Autodesk Inventor part; units mm, degrees
ref_plane "YZ Plane" through (0, 0, 0) normal (1, 0, 0) x (0, 1, 0)
ref_plane "XZ Plane" through (0, 0, 0) normal (0, 1, 0) x (-1, 0, 0)
ref_plane "XY Plane" through (0, 0, 0) normal (0, 0, 1) x (1, 0, 0)
ref_plane "工作平面1" through (0, 0, 214.75) normal (0, 0, 1) x (1, 0, 0)
sketch "草图2" plane through (0, 0, 214.75) normal (0, 0, 1) x (1, 0, 0)
  line L0 (15, -0.25) -> (15, -3.75)
  line L1 (15, 3.75) -> (15, 0.75)
  line L2 (15, 0.75) -> (13.5, 0.75)
  line L3 (13.5, 0.75) -> (13.5, -0.25)
  line L4 (13.5, -0.25) -> (15, -0.25)
  line L5 (27.5, 3.75) -> (-27.5, 3.75)
  line L6 (-15, 0.75) -> (-15, 3.75)
  line L7 (-15, -3.75) -> (-15, -0.25)
  line L8 (-13.5, 0.75) -> (-15, 0.75)
  line L9 (-13.5, -0.25) -> (-13.5, 0.75)
  line L10 (-15, -0.25) -> (-13.5, -0.25)
  line L11 (-15, -4.25) -> (15, -4.25)
  line L12 (-15, -3.75) -> (-15, -4.25)
  line L13 (15, -4.25) -> (15, -3.75)
  line L14 (18, 3.75) -> (18, -8.25)
  line L15 (-18, 3.75) -> (-18, -8.25)
  line L16 (-18, -8.25) -> (18, -8.25)
  point P0 (0, 0)
  dimension "d0" = 12
  dimension "d1" = 3
  dimension "d2" = 12
  dimension "d3" = 3
extrude "拉伸1" add sketch "草图2" along normal blind 50 contours L4 L3 L2 L1 L5 L14 L16 L15 L6 L8 L9 L10 L7 L12 L11 L13 L0
sketch "草图3" plane through (-18, -8.25, 214.75) normal (0, -1, 0) x (1, 0, 0)
  line L0 (0, 0) -> (0, 50)
  line L1 (0, 0) -> (36, 0)
  line L2 (0, 50) -> (14, 50)
  line L3 (14, 50) -> (14, 0)
  line L4 (14, 0) -> (0, 0)
  line L5 (0, 0) -> (0, 50)
  line L6 (0, 50) -> (36, 50)
  line L7 (36, 50) -> (22, 50)
  line L8 (22, 50) -> (22, 0)
  line L9 (22, 0) -> (36, 0)
  line L10 (36, 0) -> (36, 50)
  point P0 (18, -214.75)
  dimension "d6" = 14
  dimension "d7" = 14
extrude "拉伸2" add sketch "草图3" along normal blind 2 contours L0 L2 L3 L1 | L8 L6 L10 L1
sketch "草图4" plane through (-18, -10.25, 214.75) normal (0, -1, 0) x (1, 0, 0)
  line L0 (0, 50) -> (0, 0)
  line L1 (14, 50) -> (0, 50)
  line L2 (0, 0) -> (14, 0)
  line L3 (36, 50) -> (22, 50)
  line L4 (36, 0) -> (36, 50)
  line L5 (22, 0) -> (36, 0)
  point P0 (18, -214.75)
  point P1 (7, 42)
  point P2 (7, 8)
  point P3 (29, 42)
  point P4 (29, 8)
  dimension "d10" = 7
  dimension "d11" = 8
  dimension "d12" = 8
  dimension "d13" = 7
  dimension "d14" = 8
  dimension "d15" = 7
  dimension "d16" = 7
  dimension "d17" = 8
hole "孔1" at (-11, -10.25, 256.75) at (-11, -10.25, 222.75) at (11, -10.25, 256.75) at (11, -10.25, 222.75) direction (0, 1, 0) diameter 3.242 depth 3 tip angle 118
properties part number "滑块"
Read the model definition and answer for the solid it produces. Units are mm, in the model's axes. A direction names the side the tool comes from. Coordinates: 2 decimals unless noted, no trailing zeros. Loops run counter-clockwise (first coordinate to the right, second up) from the corner with the lowest first, then second, coordinate; pieces in that order, holes last. Notation, with made-up numbers: (9, -15.75) -> (23, -15.75) arc R31 ccw to (23, 20.25) -> close; hole circle Ø6 at (88, -36.5). An arc over 180 degrees is marked (long way). Return JSON: item names as keys, results as strings.
Item 1: For a pull along X with two mould halves and no side action, classify faces 6 (the flat face through (0, -5, 214.75)), 7 (the cylindrical face through (-11.07, -8.73, 224.37)), 8 (the flat face through (-15, -2, 239)) as +X half, -X half, draft (parallel to the pull), parting line (faces both ways), or undercut.
Answers:
{"face 6": "draft", "face 7": "undercut", "face 8": "undercut"}
Item 2: Find section C-C (x = 3). Determine the outline of the cut face in (y, z).
Answers:
{"outline": "(-8.25, 214.75) -> (-4.25, 214.75) -> (-4.25, 264.75) -> (-8.25, 264.75) -> close"}
Item 3: Flat-ended cylindrical pins translate along their axes: P1, Ø3, axis at x = 11, z = 222.75, coming from the +Y side; P2, Ø6, axis at x = 11, z = 252.5, coming from the +Y side; P3, Ø2, axis at x = 10.5, y = -3, coming from the +Z side. Find the tip coordinate at first contact, or state that the pin passes through.
Answers:
{"P1": "stops at y = -4.25", "P2": "stops at y = 0.75", "P3": "passes through"}
Item 4: Find section B-B (z = 231). Determine the outline of the cut face in (x, y).
Answers:
{"outline": "(-18, -10.25) -> (-4, -10.25) -> (-4, -8.25) -> (4, -8.25) -> (4, -10.25) -> (18, -10.25) -> (18, 3.75) -> (15, 3.75) -> (15, 0.75) -> (13.5, 0.75) -> (13.5, -0.25) -> (15, -0.25) -> (15, -4.25) -> (-15, -4.25) -> (-15, -0.25) -> (-13.5, -0.25) -> (-13.5, 0.75) -> (-15, 0.75) -> (-15, 3.75) -> (-18, 3.75) -> close"}
Item 5: Find the intervals of material crossed by probe 1 along X at (y, z) = (-8.9, 222.75); probe 2 along Z at (x, y) = (-11, -9); probe 3 along X at (y, z) = (-8.05, 222.75), in increasing order.
Answers:
{"probe 1": "x = -18 to -12.62, -9.38 to -4, 4 to 9.38, 12.62 to 18", "probe 2": "z = 214.75 to 221.13, 224.37 to 255.13, 258.37 to 264.75", "probe 3": "x = -18 to -12.62, -9.38 to 9.38, 12.62 to 18"}
Item 6: For faces 1 (the flat face through (15, 2, 239)), 2 (the flat face through (-14, -0.25, 239)), 3 (the cylindrical face through (10.93, -8.73, 224.37)), 4 (the flat face through (-11, -10.25, 240)), 5 (the flat face through (4, -9, 240)), determine the directions among +Z, -Z, +X, -X, +Y, -Y from which every point of the face is accessible in a straight line to the end or side of a thin tool.
Answers:
{"face 1": "+Z, -Z, +Y", "face 2": "+Z, -Z", "face 3": "-Y", "face 4": "+Z, -Z, +X, -X, -Y", "face 5": "+Z, -Z, -Y"}
Item 7: Find section D-D (x = -8.5). Determine the outline of the cut face in (y, z).
Answers:
{"outline": "(-10.25, 214.75) -> (-4.25, 214.75) -> (-4.25, 264.75) -> (-10.25, 264.75) -> close"}
Item 8: Find section A-A (y = -2.5). Determine the outline of the cut face in (x, z), plus the area to 3 significant figures.
Answers:
{"outline": "(-18, 214.75) -> (-15, 214.75) -> (-15, 264.75) -> (-18, 264.75) -> close; (15, 214.75) -> (18, 214.75) -> (18, 264.75) -> (15, 264.75) -> close", "area": "300 mm2"}
